Answer from the drawing. Dimensions are ordinates in mm from the lowest x, y and z of the part. A direction names the side the tool comes from. Round coordinates to 2 decimals unless told otherwise and drop trailing zeros. Loops run counter-clockwise (first coordinate to the right, second up) from the corner with the lowest first, then second, coordinate; pieces in that order, holes last. Notation, with made-up numbers: (-24.5, -3) - (30.5, -3) arc R19 cw to (30.5, 7) - close; hole circle Ø10 at (73.25, -28). An arc over 180 degrees is marked (long way). Return JSON: item names as keys, results as strings.
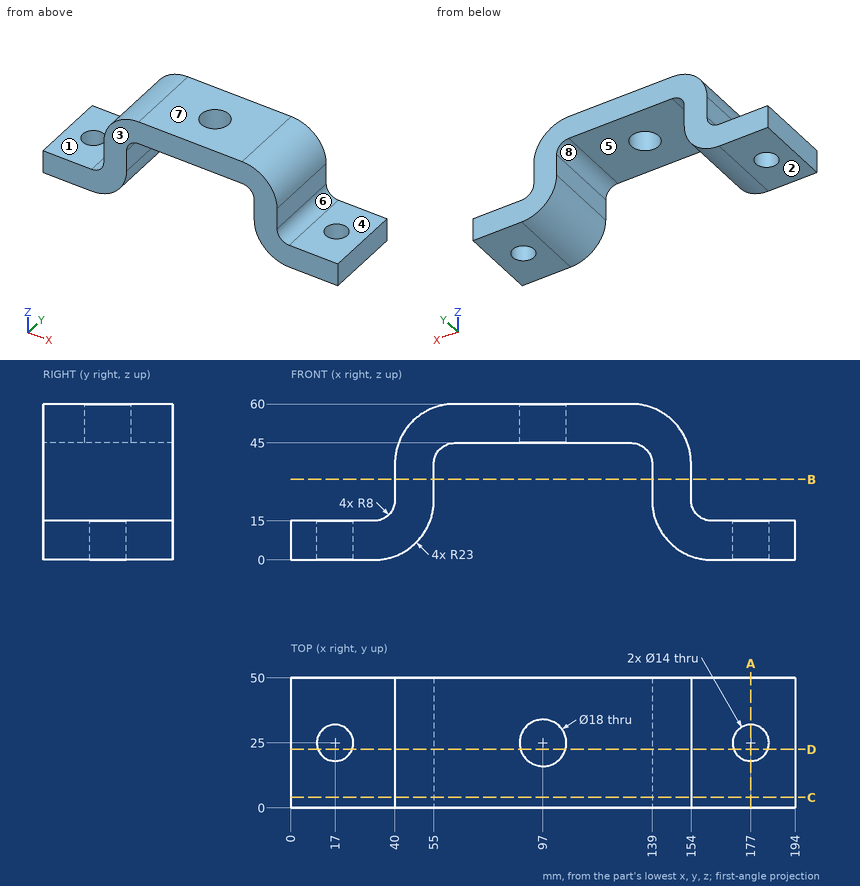
1) Section D-D (y = 22.5) is taken. Count the separate pieces of the cut face and the enclosed holes in it, and give its area (3 significant figures).
Verdict:
{"separate pieces": "4", "enclosed holes": "0", "area": "3,210 mm2"}
2) A tool of negligible diameter and unlimited length cuts with its end or side. For the marked faces 1, 2, 3, 4 and 5, from which of +Z, -Z, +X, -X, +Y, -Y can it reach the whole face along a straight path? Write none if from no direction.
Verdict:
{"face 1": "+Z, -X, +Y, -Y", "face 2": "-Z, +X, -X, +Y, -Y", "face 3": "+Z, -Z, +X, -X, -Y", "face 4": "+Z, +X, +Y, -Y", "face 5": "-Z, +Y, -Y"}
3) Find the intervals of material crossed by L1, parallel to X at y = 12.5, z = 23.5; L2, parallel to Y at x = 17, z = 4; L3, parallel to Y at x = 97, z = 55, in increasing order.
Verdict:
{"L1": "x = 40 to 55, 139 to 154", "L2": "y = 0 to 18, 32 to 50", "L3": "y = 0 to 16, 34 to 50"}
4) Determine the mould class of the marked faces 6, 7 and 8 for opening direction X: pulls with the +X half, pulls with the -X half, needs draft (parallel to the pull), parting line crosses it, or undercut.
Verdict:
{"face 6": "pulls with the +X half", "face 7": "needs draft", "face 8": "undercut"}
5) Flat-ended cylindrical pins translate along their axes: pin 1 (1.5 mm diameter, centred on x = 47.5, y = 27.5, fed in from -Z); pin 2 (16 mm diameter, centred on x = 97, y = 25, fed in from +Z); pin 3 (9.5 mm diameter, centred on x = 184, y = 20.5, fed in from +Z); pin 4 (4 mm diameter, centred on y = 16, z = 29, fed in from -X). Find the tip coordinate at first contact, or state that the pin passes through.
Verdict:
{"pin 1": "stops at z = 5.35", "pin 2": "passes through", "pin 3": "stops at z = 15", "pin 4": "stops at x = 40"}
6) Section A-A (x = 177) is taken. Give the vertices of the cut face in (y, z).
Verdict:
{"outline": "(0, 0) - (18, 0) - (18, 15) - (0, 15) - close; (32, 0) - (50, 0) - (50, 15) - (32, 15) - close"}
7) Section C-C (y = 4) is taken. Give the vertices of the cut face in (x, z).
Verdict:
{"outline": "(0, 0) - (32, 0) arc R23 ccw to (55, 23) - (55, 37) arc R8 cw to (63, 45) - (131, 45) arc R8 cw to (139, 37) - (139, 23) arc R23 ccw to (162, 0) - (194, 0) - (194, 15) - (162, 15) arc R8 cw to (154, 23) - (154, 37) arc R23 ccw to (131, 60) - (63, 60) arc R23 ccw to (40, 37) - (40, 23) arc R8 cw to (32, 15) - (0, 15) - close"}
8) Section B-B (z = 31) is taken. Give the vertices of the cut face in (x, y), and give its area (3 significant figures).
Verdict:
{"outline": "(40, 0) - (55, 0) - (55, 50) - (40, 50) - close; (139, 0) - (154, 0) - (154, 50) - (139, 50) - close", "area": "1,500 mm2"}
